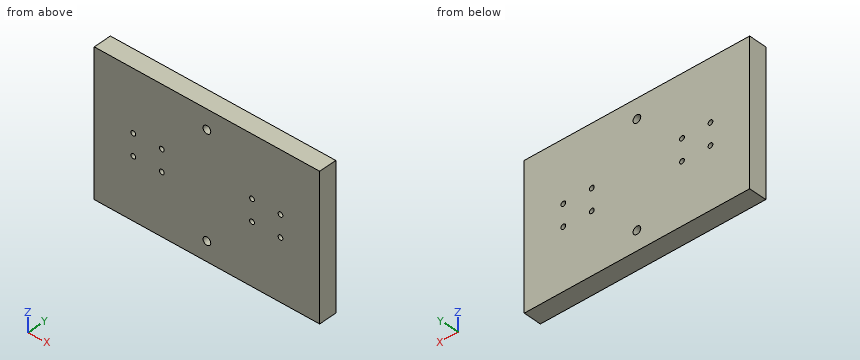
from build123d import *

# Parameters (mm, degrees)
F0_W     = 190
F0_H     = 15
F1_DEPTH = 120
F2_R     = 2
F2_R_2   = 0.903802
F2_R_3   = 1.110636
F2_R_4   = 1.007085
F3_DEPTH = 15.001
F4_R     = 3.25
F5_DEPTH = 15.001


with BuildPart() as f1:
    # F0 (on Top) → F1 (new body)
    with BuildSketch(Plane.XY):
        Rectangle(F0_W, F0_H)
    extrude(amount=F1_DEPTH)

    # F2 (on face) → F3 (cut, through all)
    with BuildSketch(Plane.XZ.offset(7.5)):
        with Locations((-62, 69)):
            Circle(F2_R)
        with Locations((-161.054239, -20.151298)):
            Circle(F2_R_2)
        with Locations((-164.950773, -26.284985)):
            Circle(F2_R_3)
        with Locations((-381.1506, -111.366101)):
            Circle(F2_R_4)
        with Locations((-38, 69)):
            Circle(F2_R)
        with Locations((-62, 51)):
            Circle(F2_R)
        with Locations((-38, 51)):
            Circle(F2_R)
        with Locations((38, 51)):
            Circle(F2_R)
        with Locations((62, 51)):
            Circle(F2_R)
        with Locations((38, 69)):
            Circle(F2_R)
        with Locations((62, 69)):
            Circle(F2_R)
    extrude(amount=-F3_DEPTH, mode=Mode.SUBTRACT)

    # F4 (on face) → F5 (cut, through all)
    with BuildSketch(Plane(origin=(0, 7.5, 0), x_dir=(-1, 0, 0), z_dir=(0, 1, 0))):
        with Locations((0, 103.75)):
            Circle(F4_R)
        with Locations((0, 16.25)):
            Circle(F4_R)
    extrude(amount=-F5_DEPTH, mode=Mode.SUBTRACT)


solid = f1.part
CAD build for the part. Positions are in the model's coordinates, mm. Give positions to 0.01 mm unless a question says otherwise; leave off trailing zeros. Write each loop counter-clockwise with the first axis right and the second up, starting at its lowest first coordinate (ties: lowest second). Pieces come first, ordered by that corner, then holes. Notation, with made-up numbers: M 82.5,2 L 93.5,2 A20 cw 93.5,28 Z; hole C 79,73.25 d5. An arc over 180 degrees is marked long. Put each result on its own line as item: value. Start each with the question number.
(1) Band-saw the part on B-B, the plane x = 0. Write the cut outline in (y, z).
(2) Probe L1, parallel to Z at x = -38, y = 0; L2, parallel to Z at x = 0, y = 1.75; L3, parallel to X at y = 3, z = 49.5. List the from-to ranges inside material, lowest first.
(3) Flat gauge pin, fed straight in: pin 1 Ø3.5 at (x, z) = (-62, 51) entering from +Y. Where does the tip first touch, or does it go through?
(4) Band-saw the part on A-A, the plane z = 69. Write the cut outline in (x, y).
(5) Band-saw the part on C-C, the plane z = 16.25. Write the cut outline in (x, y), and give its area (3 significant figures).
(6) Band-saw the part on D-D, the plane x = -38. Write the cut outline in (y, z).
Response values:
1. outline: M -7.5,0 L 7.5,0 L 7.5,13 L -7.5,13 Z; M -7.5,19.5 L 7.5,19.5 L 7.5,100.5 L -7.5,100.5 Z; M -7.5,107 L 7.5,107 L 7.5,120 L -7.5,120 Z
2. L1: z = 0 to 49, 53 to 67, 71 to 120
2. L2: z = 0 to 13, 19.5 to 100.5, 107 to 120
2. L3: x = -95 to -63.32, -60.68 to -39.32, -36.68 to 36.68, 39.32 to 60.68, 63.32 to 95
3. pin 1: passes through
4. outline: M -95,-7.5 L -64,-7.5 L -64,7.5 L -95,7.5 Z; M -60,-7.5 L -40,-7.5 L -40,7.5 L -60,7.5 Z; M -36,-7.5 L 36,-7.5 L 36,7.5 L -36,7.5 Z; M 40,-7.5 L 60,-7.5 L 60,7.5 L 40,7.5 Z; M 64,-7.5 L 95,-7.5 L 95,7.5 L 64,7.5 Z
5. outline: M -95,-7.5 L -3.25,-7.5 L -3.25,7.5 L -95,7.5 Z; M 3.25,-7.5 L 95,-7.5 L 95,7.5 L 3.25,7.5 Z
5. area: 2,750 mm2
6. outline: M -7.5,0 L 7.5,0 L 7.5,49 L -7.5,49 Z; M -7.5,53 L 7.5,53 L 7.5,67 L -7.5,67 Z; M -7.5,71 L 7.5,71 L 7.5,120 L -7.5,120 Z
